Drawing for the job (mm, zero at the part's lowest x, y, z). A direction names the side the tool comes from. Coordinates: 2 decimals unless noted, no trailing zeros. Loops run counter-clockwise (first coordinate to the right, second up) from the corner with the lowest first, then second, coordinate; pieces in that order, holes last. Notation, with made-up numbers: (29.5, -39) - (87.5, -39) arc R13 ccw to (87.5, -23) - close; hole circle Ø7 at (14.5, 63). An arc over 180 degrees is marked (long way). One line per item, written item: value.
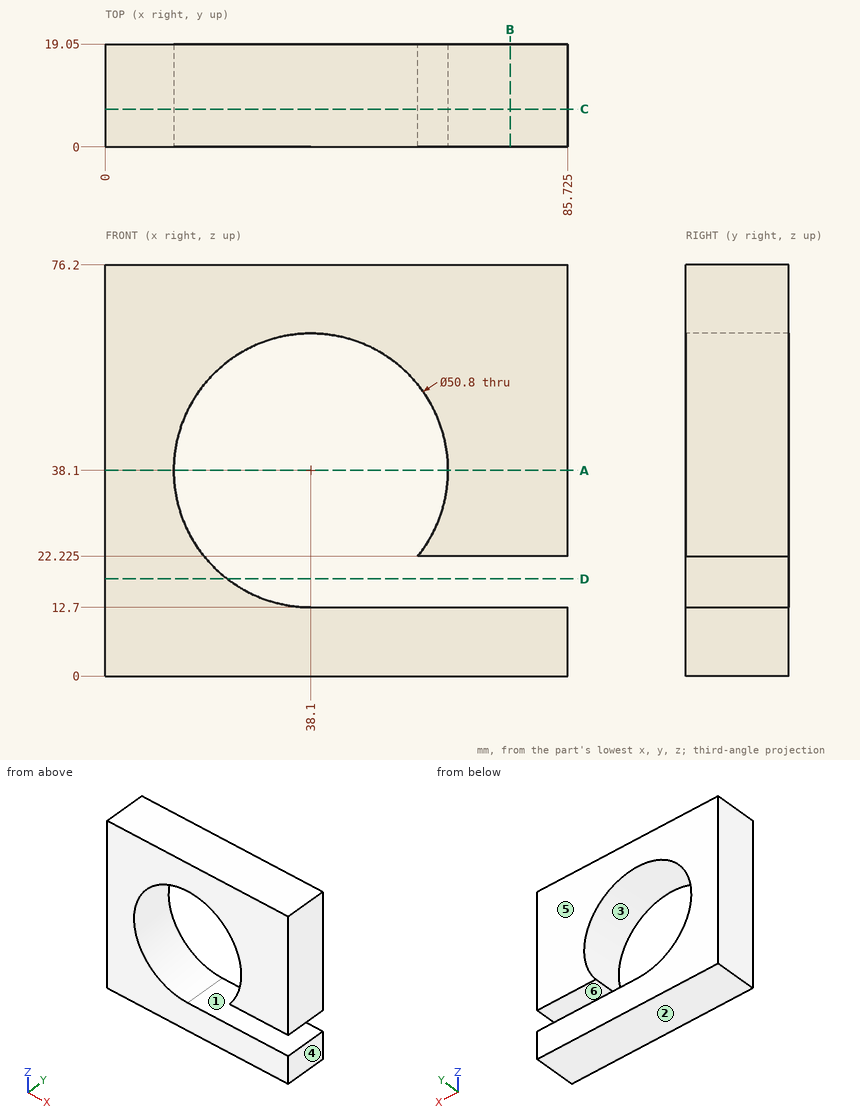
Item 1: Cut at A-A, the plane z = 38.1. Write the cut outline in (x, y) (3 decimals), then the cut area to 3 significant figures.
Check result:
outline: (0, 0) - (12.7, 0) - (12.7, 19.05) - (0, 19.05) - close; (63.5, 0) - (85.725, 0) - (85.725, 19.05) - (63.5, 19.05) - close
area: 665 mm^2
Item 2: Probe probe 1 along X at (y, z) = (10.5, 38.1) (3 decimals); probe 2 along Z at (x, y) = (61.5, 1.5) (3 decimals); probe 3 along Z at (x, y) = (38.1, 11). List the from-to ranges inside material, lowest first. Write a range as from..to.
Check result:
probe 1: x = 0..12.7, 63.5..85.725
probe 2: z = 0..12.7, 22.225..28.221, 47.979..76.2
probe 3: z = 0..12.7, 63.5..76.2
Item 3: Cut at D-D, the plane z = 18. Write the cut outline in (x, y), then the cut area to 3 significant figures.
Check result:
outline: (0, 0) - (22.57, 0) - (22.57, 19.05) - (0, 19.05) - close
area: 430 mm^2
Item 4: Cut at C-C, the plane y = 7. Write the cut outline in (x, z) (3 decimals).
Check result:
outline: (0, 0) - (85.725, 0) - (85.725, 12.7) - (38.1, 12.7) arc R25.4 cw (long way) to (57.928, 22.225) - (85.725, 22.225) - (85.725, 76.2) - (0, 76.2) - close
Item 5: Tool access for the marked faces 5 and 6: list every direction of +Z, -Z, +X, -X, +Y, -Y with a clear straight run to the whole face (end or side of a thin tool).
Check result:
face 5: +Z, -Z, +X, -X, +Y
face 6: +X, +Y, -Y
Item 6: Cut at B-B, the plane x = 75. Write the cut outline in (y, z) (3 decimals).
Check result:
outline: (0, 0) - (19.05, 0) - (19.05, 12.7) - (0, 12.7) - close; (0, 22.225) - (19.05, 22.225) - (19.05, 76.2) - (0, 76.2) - close
Item 7: Pull direction Z, two halves, no side cores. Call the marked faces 1, 2, 3 and 4: released by +Z, released by -Z, zero draft, split by the parting line, or undercut.
Check result:
face 1: undercut
face 2: released by -Z
face 3: undercut
face 4: zero draft
